Geometry check sheet. Reference: drawing and pictorial views, mm from the part's lowest x, y, z. A direction names the side the tool comes from. Coordinates: 2 decimals unless noted, no trailing zeros. Write each loop counter-clockwise with the first axis right and the second up, starting at its lowest first coordinate (ties: lowest second). Pieces come first, ordered by that corner, then holes. Notation, with made-up numbers: M -11,-7.5 L 21,-7.5 A19 cw 21,3.5 Z; hole C 82,64 d10. An arc over 180 degrees is marked long. One line per item, written item: value.
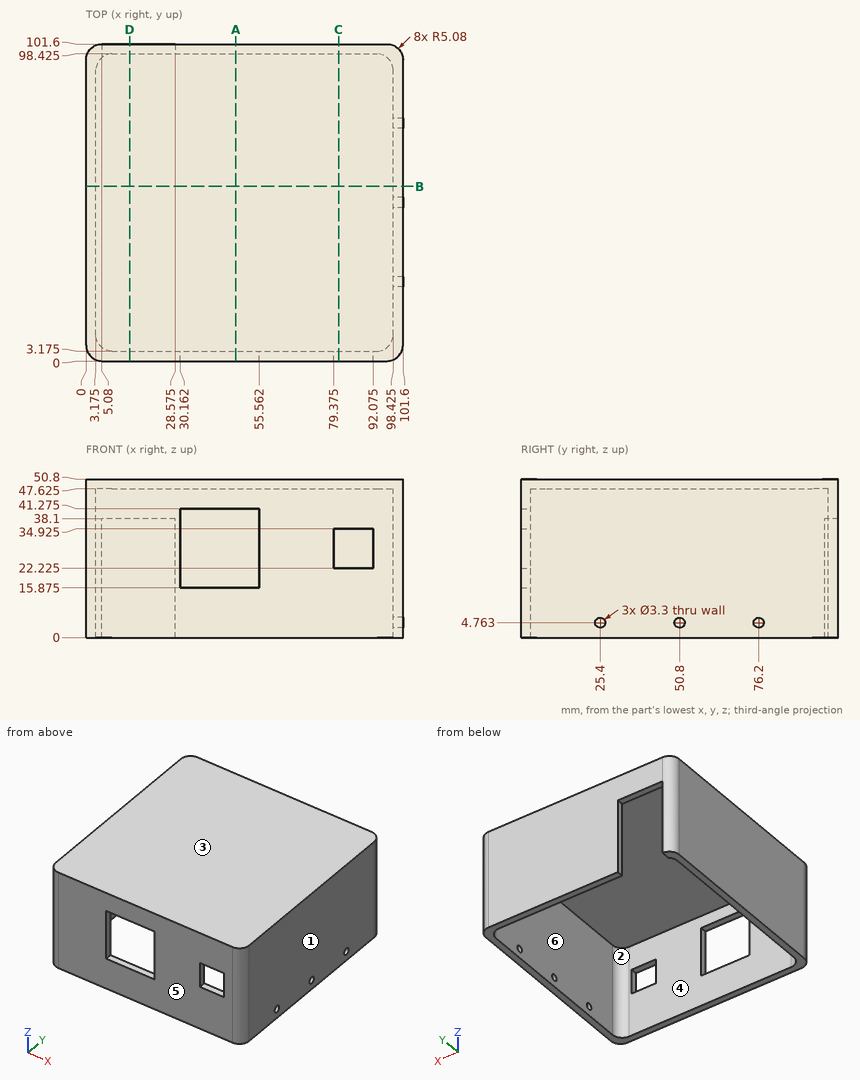
Item 1: Draft check along Y on the marked faces 3, 4, 5 and 6. Enter one of: released by +Y, released by -Y, zero draft, split by the parting line, or undercut.
The answers:
face 3: zero draft
face 4: undercut
face 5: released by -Y
face 6: undercut
Item 2: Go/stop test with flat-tipped pins: P1, Ø2, axis at x = 27.5, z = 34, coming from the +Y side (1 decimal); P2, Ø2.5, axis at x = 87, y = 2, coming from the -Z side; P3, Ø2.5, axis at y = 76.2, z = 4.76, coming from the +X side (1 decimal); P4, Ø1.6, axis at y = 2, z = 31, coming from the +X side. Record where each tip stops, or that it passes through.
The answers:
P1: stops at y = 3.2
P2: stops at z = 0
P3: stops at x = 3.2
P4: stops at x = 101.06
Item 3: Cross-section at A-A, the plane x = 48. Enter the section's corners in (y, z) (1 decimal).
The answers:
outline: M 0,0 L 3.2,0 L 3.2,15.9 L 0,15.9 Z; M 0,41.3 L 3.2,41.3 L 3.2,47.6 L 98.4,47.6 L 98.4,0 L 101.6,0 L 101.6,50.8 L 0,50.8 Z
Item 4: Scan lines: line 1 (Z direction, x = 100.2, y = 50.8); line 2 (X direction, y = 89, z = 23) (1 decimal). Record each from-to range of solid material in increasing order.
The answers:
line 1: z = 0 to 3.11, 6.41 to 50.8
line 2: x = 0 to 3.2, 98.4 to 101.6
Item 5: Cross-section at D-D, the plane x = 14. Enter the section's corners in (y, z) (1 decimal), and give its area (3 significant figures).
The answers:
outline: M 0,0 L 3.2,0 L 3.2,47.6 L 98.4,47.6 L 98.4,38.1 L 101.6,38.1 L 101.6,50.8 L 0,50.8 Z
area: 504 mm²
Item 6: Cross-section at B-B, the plane y = 56. Enter the section's corners in (x, z) (1 decimal), and give its area (3 significant figures).
The answers:
outline: M 0,0 L 3.2,0 L 3.2,47.6 L 98.4,47.6 L 98.4,0 L 101.6,0 L 101.6,50.8 L 0,50.8 Z
area: 625 mm²
Item 7: Access from +Z, -Z, +X, -X, +Y, -Y to the whole of each face (thin tool, end or side, straight path). Record for the marked faces 1 and 2.
The answers:
face 1: +Z, -Z, +X, +Y, -Y
face 2: -Z
Item 8: Cross-section at C-C, the plane x = 81. Enter the section's corners in (y, z) (1 decimal).
The answers:
outline: M 0,0 L 3.2,0 L 3.2,22.2 L 0,22.2 Z; M 0,34.9 L 3.2,34.9 L 3.2,47.6 L 98.4,47.6 L 98.4,0 L 101.6,0 L 101.6,50.8 L 0,50.8 Z
